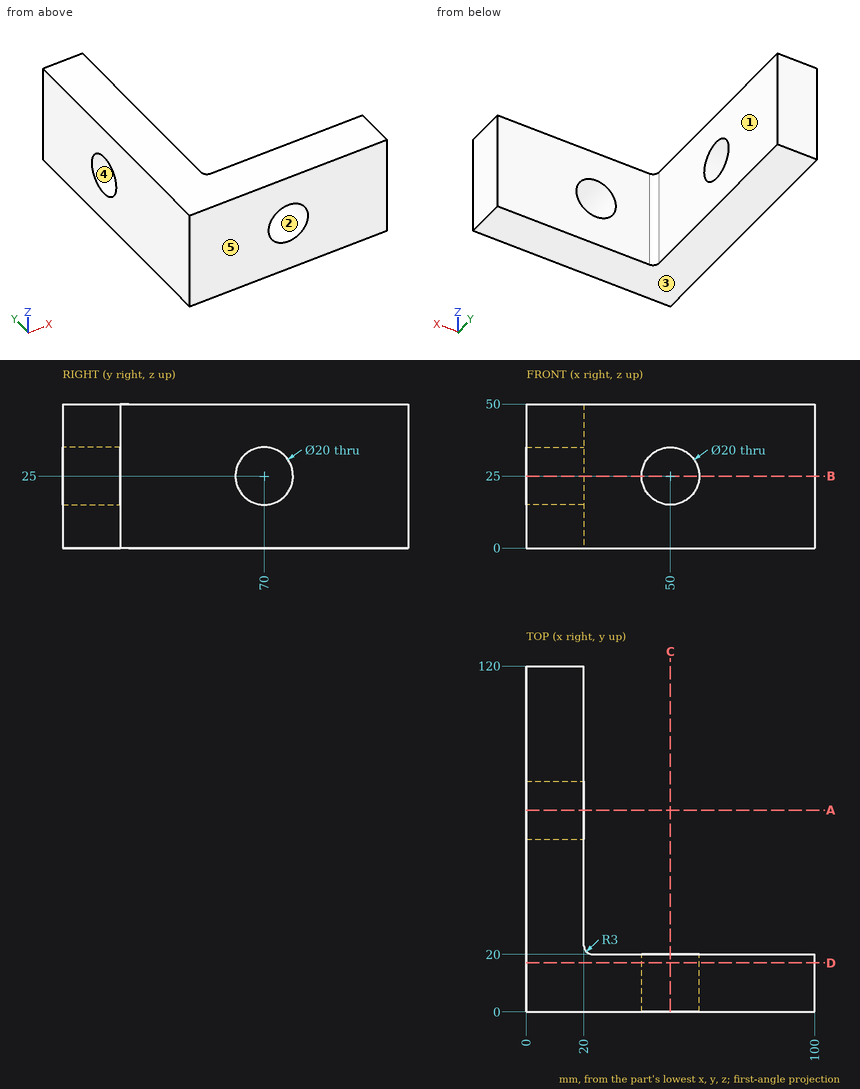
Can you work these out from the drawing? Everything is in mm from the part's minimum corner. A direction names the side the tool comes from. Round coordinates to 2 decimals unless told otherwise and drop trailing zeros. Write each loop counter-clockwise with the first axis right and the second up, starting at its lowest first coordinate (ties: lowest second). Pieces come first, ordered by that corner, then holes. Notation, with made-up numbers: (3.25, 47) - (45.25, 47) arc R10 cw to (45.25, 58) - close; hole circle Ø9 at (40.25, 67). An arc over 180 degrees is marked (long way). Write each question's results on one line, items separated by ' | '. Start each with the question number.
1) Suppose I cut it at A-A (y = 70). List the corners of the cut face in (x, z) for me.
2) Please list where these lines run through material, in increasing order: line 1 (X direction, y = 6, z = 25); line 2 (Y direction, x = 7, z = 25); line 3 (X direction, y = 44, z = 23).
3) Which directions (+Z, -Z, +X, -X, +Y, -Y) give clear straight access to the entire face, cutting with the end or side of a thin tool? Please do the marked faces 1 and 2.
4) We'd pull the mould along Z, two halves only. Please class the marked faces 3, 4 and 5: released by +Z, released by -Z, zero draft, split by the parting line, or undercut.
5) Suppose I cut it at B-B (z = 25). List the corners of the cut face in (x, y) for me.
6) For pin 1 Ø18 at (y, z) = (70, 25) entering from +X; pin 2 Ø10 at (x, z) = (90, 31) entering from +Y; pin 3 Ø15 at (y, z) = (68, 28.5) entering from +X, each with a flat end and sliding along its axis, tell me the tip position at first contact or that it passes through.
7) Suppose I cut it at D-D (y = 17). List the corners of the cut face in (x, z) for me.
Here are the results:
1) outline: (0, 0) - (20, 0) - (20, 15) - (0, 15) - close; (0, 35) - (20, 35) - (20, 50) - (0, 50) - close
2) line 1: x = 0 to 40, 60 to 100 | line 2: y = 0 to 60, 80 to 120 | line 3: x = 0 to 20
3) face 1: +Z, -Z, +X, +Y | face 2: +Y, -Y
4) face 3: released by -Z | face 4: undercut | face 5: zero draft
5) outline: (0, 0) - (40, 0) - (40, 20) - (23, 20) arc R3 cw to (20, 23) - (20, 60) - (0, 60) - close; (0, 80) - (20, 80) - (20, 120) - (0, 120) - close; (60, 0) - (100, 0) - (100, 20) - (60, 20) - close
6) pin 1: passes through | pin 2: stops at y = 20 | pin 3: stops at x = 20
7) outline: (0, 0) - (100, 0) - (100, 50) - (0, 50) - close; hole circle Ø20 at (50, 25)
